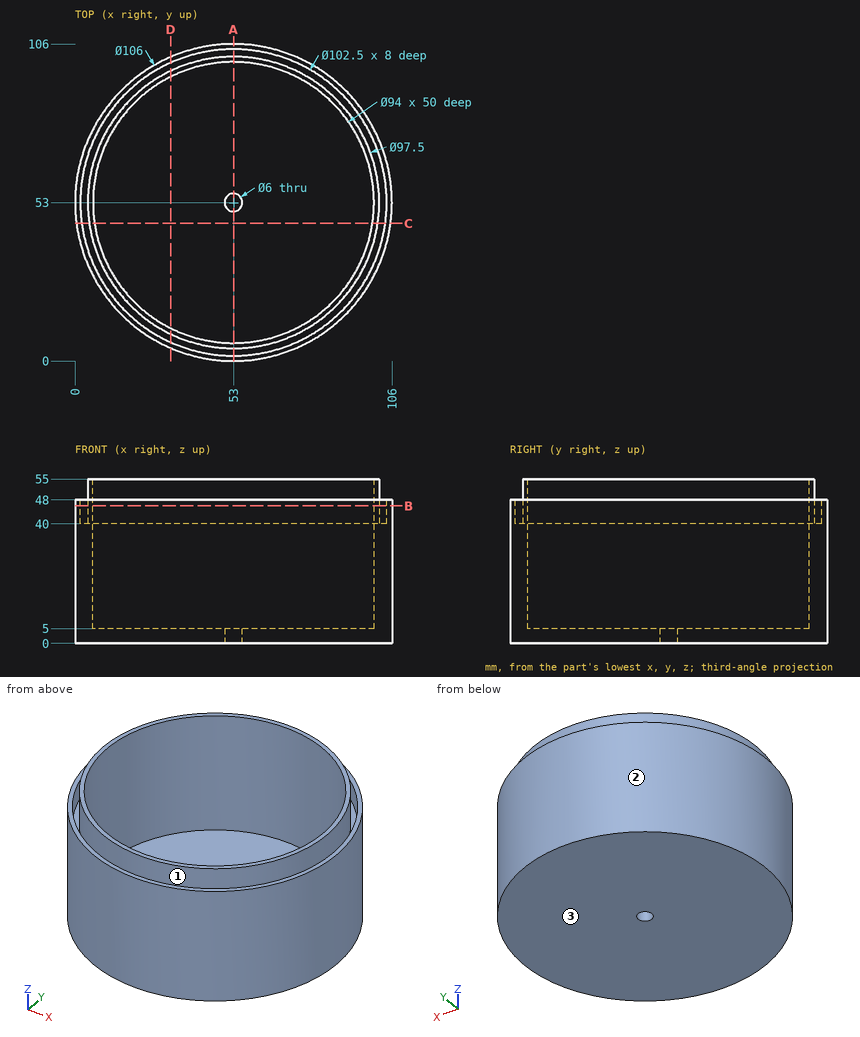
Job drawing, mm, ordinate dimensions from the low corner. One solid piece. Give positions to 0.01 mm unless a question says otherwise; leave off trailing zeros. Loops run counter-clockwise (first coordinate to the right, second up) from the corner with the lowest first, then second, coordinate; pieces in that order, holes last. Notation, with made-up numbers: M 35.5,-9 L 80.5,-9 A7 ccw 80.5,-3 Z; hole C 82.5,33 d9. An arc over 180 degrees is marked long. Answer in a Markdown table with one row per item. Add a question column.
Item 1: Drop flat-ended pins along their axis: P1, Ø2, axis at x = 84, z = 10.5, coming from the +Y side; P2, Ø3, axis at y = 11.5, z = 47.5, coming from the +X side; P3, Ø5, axis at y = 77.5, z = 21.5, coming from the -X side. Give the stop position or say it passes through.
Item 2: Band-saw the part on B-B on z = 46. Give the cut face in (x, y).
Item 3: Mould opens along X. For the marked faces 1, 2 and 3 say: +X half, -X half, draft (parallel to the pull), parting line (faces both ways), or undercut.
Item 4: Band-saw the part on D-D on x = 32. Give the cut face in (y, z), then the cut area to 3 significant figures.
Item 5: Band-saw the part on A-A on x = 53. Give the cut face in (y, z).
Item 6: Band-saw the part on C-C on y = 46. Give the cut face in (x, z).
Item 7: Probe probe 1 along X at (y, z) = (83.5, 41.5); probe 2 along Y at (x, z) = (27, 42); probe 3 along Y at (x, z) = (85, 44). List the from-to ranges inside material, lowest first.
Reply:
| question | item | result |
|---|---|---|
| 1 | P1 | stops at y = 96.69 |
| 1 | P2 | stops at x = 87.77 |
| 1 | P3 | stops at x = 4.78 |
| 2 | outline | C 53,53 d106; C 53,53 d97.5; hole C 53,53 d102.5; hole C 53,53 d94 |
| 3 | face 1 | undercut |
| 3 | face 2 | parting line |
| 3 | face 3 | draft |
| 4 | outline | M 4.34,0 L 101.66,0 L 101.66,48 L 99.75,48 L 99.75,40 L 97,40 L 97,55 L 95.05,55 L 95.05,5 L 10.95,5 L 10.95,55 L 9,55 L 9,40 L 6.25,40 L 6.25,48 L 4.34,48 Z |
| 4 | area | 1,040 mm^2 |
| 5 | outline | M 0,0 L 50,0 L 50,5 L 6,5 L 6,55 L 4.25,55 L 4.25,40 L 1.75,40 L 1.75,48 L 0,48 Z; M 56,0 L 106,0 L 106,48 L 104.25,48 L 104.25,40 L 101.75,40 L 101.75,55 L 100,55 L 100,5 L 56,5 Z |
| 6 | outline | M 0.46,0 L 105.54,0 L 105.54,48 L 103.77,48 L 103.77,40 L 101.24,40 L 101.24,55 L 99.48,55 L 99.48,5 L 6.52,5 L 6.52,55 L 4.76,55 L 4.76,40 L 2.23,40 L 2.23,48 L 0.46,48 Z |
| 7 | probe 1 | x = 9.66 to 11.81, 14.97 to 17.24, 88.76 to 91.03, 94.19 to 96.34 |
| 7 | probe 2 | y = 6.82 to 8.83, 11.76 to 13.85, 92.15 to 94.24, 97.17 to 99.18 |
| 7 | probe 3 | y = 10.75 to 12.97, 16.22 to 18.58, 87.42 to 89.78, 93.03 to 95.25 |
